Autodesk Inventor part; units mm, degrees
ref_plane "YZ Plane" through (0, 0, 0) normal (1, 0, 0) x (0, 1, 0)
ref_plane "XZ Plane" through (0, 0, 0) normal (0, 1, 0) x (-1, 0, 0)
ref_plane "XY Plane" through (0, 0, 0) normal (0, 0, 1) x (1, 0, 0)
sketch "Sketch1" plane through (0, 0, 0) normal (0, 0, 1) x (1, 0, 0)
  circle A0 centre (0, 0) radius 25.4
  dimension "d0" = 50.8
extrude "Extrusion1" add sketch "Sketch1" along normal blind 101.6
sketch "Sketch2" plane through (0, 0, 0) normal (0, 0, 1) x (1, 0, 0)
  line L0 (88.9, 38.1) -> (-88.9, 38.1)
  line L1 (-88.9, 38.1) -> (-88.9, -38.1)
  line L2 (-88.9, -38.1) -> (88.9, -38.1)
  line L3 (88.9, -38.1) -> (88.9, 38.1)
  point P0 (0, 0)
  point P1 (0, 38.1)
  point P2 (88.9, 0)
  dimension "d3" = 76.2
  dimension "d4" = 177.8
extrude "Extrusion2" add sketch "Sketch2" against normal blind 999.998
properties part number "solid_for_CFD_test_06(testing device)"
Design review of the part built by this model. Coordinates are the model's own, in mm. A direction names the side the tool comes from. Coordinates: 2 decimals unless noted, no trailing zeros. Write each loop counter-clockwise with the first axis right and the second up, starting at its lowest first coordinate (ties: lowest second). Pieces come first, ordered by that corner, then holes.
1) Add section B-B (x = 0). Write out the cut boundary in (y, z), plus the area to 3 significant figures.
2) Add section C-C (x = 72.5). Write out the cut boundary in (y, z).
3) Machinability: for faces 1 (the flat face through (0, 0, 101.6)), 2 (the cylindrical face through (-5.506, 24.796, 50.089)), which of the approach directions +Z, -Z, +X, -X, +Y, -Y give a long, thin tool a straight path to every point of the face, cutting with its end or side? Answer none if there is none.
4) Add section A-A (y = 0). Write out the cut boundary in (x, z), plus the area to 3 significant figures.
5) To check wall thickness, follow L1, parallel to Z at x = 53.5, y = 12. State the ranges of the line that lie inside material, in increasing order.
Check result:
1. outline: (-38.1, -1000) - (38.1, -1000) - (38.1, 0) - (25.4, 0) - (25.4, 101.6) - (-25.4, 101.6) - (-25.4, 0) - (-38.1, 0) - close
1. area: 81,400 mm2
2. outline: (-38.1, -1000) - (38.1, -1000) - (38.1, 0) - (-38.1, 0) - close
3. face 1: +Z, +X, -X, +Y, -Y
3. face 2: +Z
4. outline: (-88.9, -1000) - (88.9, -1000) - (88.9, 0) - (25.4, 0) - (25.4, 101.6) - (-25.4, 101.6) - (-25.4, 0) - (-88.9, 0) - close
4. area: 183,000 mm2
5. L1: z = -1000 to 0
